Design review of the part built by this model. Coordinates are the model's own, in mm. Face numbers are marked on the shaded views. A direction names the side the tool comes from. Give positions to 0.01 mm unless a question says otherwise; leave off trailing zeros. Write each loop counter-clockwise with the first axis right and the second up, starting at its lowest first coordinate (ties: lowest second). Pieces come first, ordered by that corner, then holes. Notation, with made-up numbers: (5, 49.5) -> (27, 49.5) arc R22 cw to (27, 61.5) -> close; hole circle Ø7 at (-35.5, -3). An arc over 180 degrees is marked (long way). Use CSV: the item, a comma, the result in double quotes.
```python
from build123d import *

# Parameters (mm, degrees)
SKETCH1_W           = 38.1
SKETCH1_H           = 25.4
SKETCH1_R           = 3.2639
BOSS_EXTRUDE1_DEPTH = 6.35
BOSS_EXTRUDE2_START = -6.35
BOSS_EXTRUDE2_DEPTH = 6.35
FILLET1_R           = 6.35
FILLET2_R           = 12.7


with BuildPart() as part:
    # Sketch1 → Boss-Extrude1 (new body)
    # profile 1 of 2: a face of its own
    with BuildSketch(Plane(origin=(0, 0, 0), x_dir=(1, 0, 0), z_dir=(0, 1, 0))):
        with Locations((0, 6.35)):
            Rectangle(SKETCH1_W, SKETCH1_H)
        with Locations(Location((-9.525, 6.35, 0), (0, 0, 270))):
            Circle(SKETCH1_R, mode=Mode.SUBTRACT)
        with Locations(Location((9.525, 6.35, 0), (0, 0, 270))):
            Circle(SKETCH1_R, mode=Mode.SUBTRACT)
    # profile 2 of 2: a face of its own
    with BuildSketch(Plane(origin=(0, 0, 0), x_dir=(1, 0, 0), z_dir=(0, 1, 0))):
        with BuildLine():
            Line((19.05, -6.35), (-19.05, -6.35))
            Line((-19.05, -6.35), (-19.05, -19.05))
            Line((-19.05, -19.05), (-4.121852568, -19.05))
            ThreePointArc((-4.121852568, -19.05), (-0.053223596, -19.377978576), (3.910332689, -20.35344423))
            Line((3.910332689, -20.35344423), (19.05, -25.4))
            Line((19.05, -25.4), (19.05, -19.05))
            Line((19.05, -19.05), (19.05, -6.35))
        make_face()
    extrude(amount=BOSS_EXTRUDE1_DEPTH)

    # Sketch1_7 → Boss-Extrude2 (add)
    with BuildSketch(Plane(origin=(0, 0, 0), x_dir=(1, 0, 0), z_dir=(0, 1, 0)).offset(BOSS_EXTRUDE2_START)):
        with BuildLine():
            Line((19.05, -6.35), (-19.05, -6.35))
            Line((-19.05, -6.35), (-19.05, -19.05))
            Line((-19.05, -19.05), (-4.121852568, -19.05))
            ThreePointArc((-4.121852568, -19.05), (-0.053223596, -19.377978576), (3.910332689, -20.35344423))
            Line((3.910332689, -20.35344423), (19.05, -25.4))
            Line((19.05, -25.4), (19.05, -19.05))
            Line((19.05, -19.05), (19.05, -6.35))
        make_face()
    extrude(amount=BOSS_EXTRUDE2_DEPTH)

    # Fillet1
    fillet1_edges = [part.edges().sort_by_distance(p)[0] for p in [
        (-19.05, 0, 19.05),
    ]]
    fillet(fillet1_edges, radius=FILLET1_R)

    # Fillet2
    fillet2_edges = [part.edges().sort_by_distance(p)[0] for p in [
        (-19.05, 3.175, -19.05),
        (19.05, 3.175, -19.05),
    ]]
    fillet(fillet2_edges, radius=FILLET2_R)


solid = part.part
```
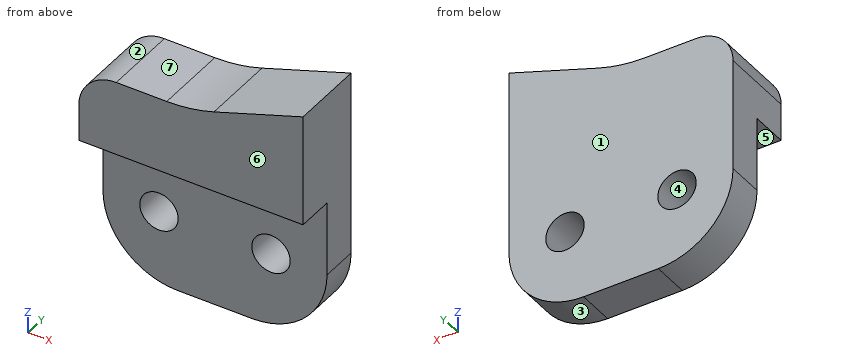
(1) Mouldability with a two-part tool opening along X and no side actions: class the marked faces 1, 2, 3 and 4 as +X half, -X half, draft (parallel to the pull), parting line (faces both ways), or undercut.
Established:
face 1,"draft"
face 2,"-X half"
face 3,"+X half"
face 4,"undercut"
(2) For line 1 along X through (y, z) = (2.25, -6.35); line 2 along X through (y, z) = (2, -8); line 3 along Z through (x, y) = (-13, -5.5), list the stretches that pass through material, from the lowest coordinate up. Write a range as [from, to].
Established:
line 1,"x = [-19.05, -12.79], [-6.26, 6.26], [12.79, 19.05]"
line 2,"x = [-18.94, -12.34], [-6.71, 6.71], [12.34, 18.94]"
line 3,"z = [6.35, 19.04]"
(3) Clearance check with flat-ended pins moving along their axes: pin 1 (6 mm diameter, centred on y = 3, z = -10.5, fed in from -X); pin 2 (20.5 mm diameter, centred on x = 1.5, z = -10.5, fed in from -Y); pin 3 (4 mm diameter, centred on y = 4.5, z = -11, fed in from +X). State where each tip first meets the part, or that it passes through.
Established:
pin 1,"stops at x = -19"
pin 2,"stops at y = 0"
pin 3,"stops at x = 18.77"
(4) Take a section at A-A (x = 12). Write out the cut boundary in (y, z).
Established:
outline,"(-6.35, 6.35) -> (0, 6.35) -> (0, -4.22) -> (6.35, -4.22) -> (6.35, 23.05) -> (-6.35, 23.05) -> close; (0, -17.72) -> (6.35, -17.72) -> (6.35, -8.48) -> (0, -8.48) -> close"
(5) Take a section at C-C (y = 4.5). Write out the cut boundary in (x, z) (3 decimals), then the cut area to 3 significant figures.
Established:
outline,"(-19.05, -6.35) arc R12.7 ccw to (-6.35, -19.05) -> (6.35, -19.05) arc R12.7 ccw to (19.05, -6.35) -> (19.05, 25.4) -> (3.91, 20.353) arc R25.4 cw to (-4.122, 19.05) -> (-12.7, 19.05) arc R6.35 ccw to (-19.05, 12.7) -> close; hole circle Ø6.528 at (-9.525, -6.35); hole circle Ø6.528 at (9.525, -6.35)"
area,"1,370 mm2"
(6) Tool access review of the marked faces 5, 6 and 7: name each direction out of +Z, -Z, +X, -X, +Y, -Y from which nothing blocks a thin tool from reaching the whole face with its end or side.
Established:
face 5,"-Z, +X, -X, -Y"
face 6,"+Z, -Z, +X, -X, -Y"
face 7,"+Z, -X, +Y, -Y"
(7) Take a section at D-D (z = 22). Write out the cut boundary in (x, y), then the cut area to 3 significant figures.
Established:
outline,"(8.85, -6.35) -> (19.05, -6.35) -> (19.05, 6.35) -> (8.85, 6.35) -> close"
area,"130 mm2"
(8) Take a section at B-B (y = -5). Write out the cut boundary in (x, z).
Established:
outline,"(-19.05, 6.35) -> (19.05, 6.35) -> (19.05, 25.4) -> (3.91, 20.35) arc R25.4 cw to (-4.12, 19.05) -> (-12.7, 19.05) arc R6.35 ccw to (-19.05, 12.7) -> close"
